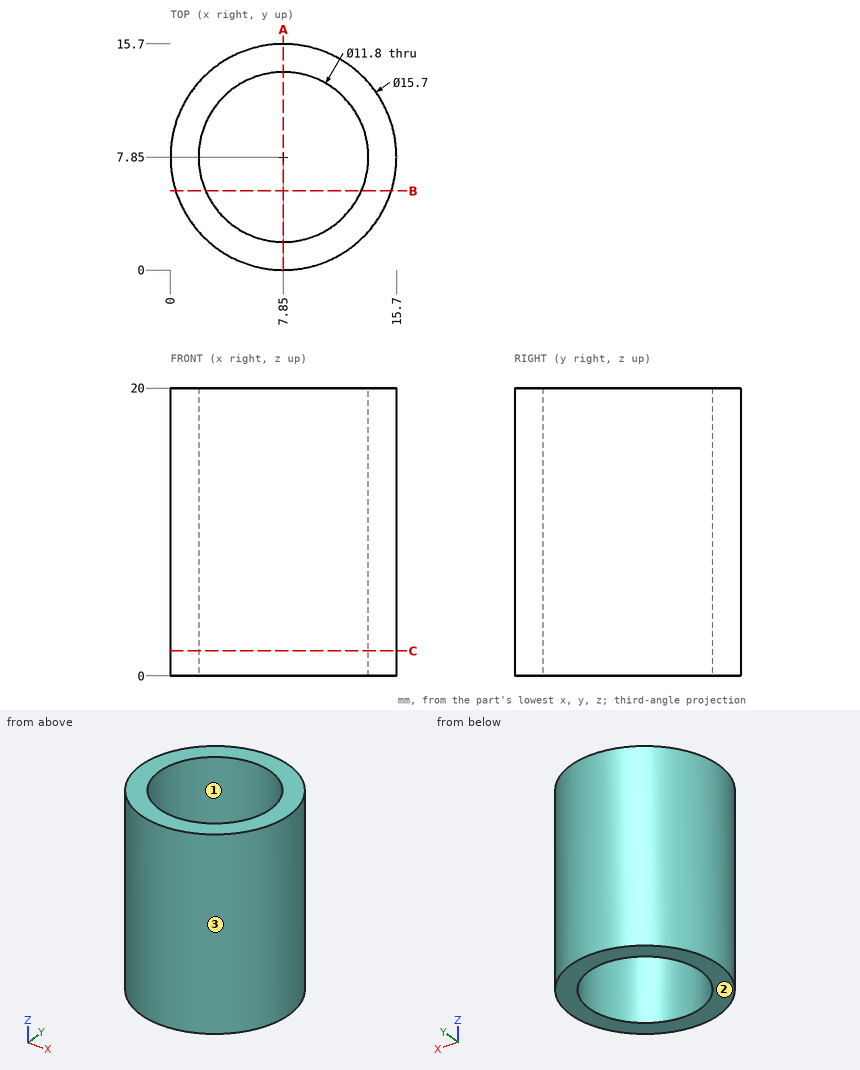
Verification items for this drawing (mm, ordinates from the low corner). Coordinates: 2 decimals unless noted, no trailing zeros. Write each loop counter-clockwise with the first axis right and the second up, starting at its lowest first coordinate (ties: lowest second). Pieces come first, ordered by that corner, then holes. Notation, with made-up numbers: M -22,39 L -2,39 A20 ccw -2,56 Z; hole C 19,3.5 d11. An arc over 180 degrees is marked long. One line per item, written item: value. Start each with the question number.
(1) Scan lines: line 1 along Y through (x, z) = (7.85, 14.5); line 2 along Y through (x, z) = (10, 6.5); line 3 along X through (y, z) = (9, 11.25). Record each from-to range of solid material in increasing order. Write a range as [from, to].
(2) Sectioned sample at A-A, the plane x = 7.85. Enter the section's corners in (y, z).
(3) Depth check by flat-ended pin: pin 1 (3 mm diameter, centred on y = 5.5, z = 16, fed in from +X); pin 2 (5 mm diameter, centred on y = 11.5, z = 7, fed in from +X); pin 3 (1 mm diameter, centred on x = 4.5, z = 16.5, fed in from -Y). Enter the tip coordinate at first touch or a pass-through.
(4) Release check for a two-part mould opening along X. For the marked faces 1, 2 and 3 record: released by +X, released by -X, zero draft, split by the parting line, or undercut.
(5) Sectioned sample at C-C, the plane z = 1.75. Enter the section's corners in (x, y), and give its area (3 significant figures).
(6) Sectioned sample at B-B, the plane y = 5.5. Enter the section's corners in (x, z).
Filled sheet:
1. line 1: [0, 1.95], [13.75, 15.7]
1. line 2: [0.3, 2.36], [13.34, 15.4]
1. line 3: [0.08, 2.06], [13.64, 15.62]
2. outline: M 0,0 L 1.95,0 L 1.95,20 L 0,20 Z; M 13.75,0 L 15.7,0 L 15.7,20 L 13.75,20 Z
3. pin 1: x = 15.65
3. pin 2: x = 15.62
3. pin 3: y = 0.54
4. face 1: undercut
4. face 2: zero draft
4. face 3: split by the parting line
5. outline: C 7.85,7.85 d15.7; hole C 7.85,7.85 d11.8
5. area: 84.2 mm²
6. outline: M 0.36,0 L 2.44,0 L 2.44,20 L 0.36,20 Z; M 13.26,0 L 15.34,0 L 15.34,20 L 13.26,20 Z
